Could you check a few things on this drawing? It's one solid part, dimensions in mm from its lowest x, y, z. A direction names the side the tool comes from. Give positions to 0.01 mm unless a question says otherwise; leave off trailing zeros. Loops run counter-clockwise (first coordinate to the right, second up) from the corner with the lowest first, then second, coordinate; pieces in that order, holes last.
1. I need wall thicknesses on line 1 along Z through (x, y) = (17.5, 22.75); line 2 along X through (y, z) = (18.25, 76.5) (1 decimal); line 3 along Y through (x, z) = (36.5, 49). Which ranges of each line are inside material? Lowest first, please.
2. Imagine slicing it at C-C (z = 34). List the corners of the cut face in (x, y) for me (1 decimal).
3. For P1, Ø3, axis at x = 61, z = 55.5, coming from the -Y side, with a flat end and sliding along its axis, tell me the tip position at first contact or that it passes through.
4. Imagine slicing it at B-B (y = 21). List the corners of the cut face in (x, z) for me (1 decimal), plus the area to 3 significant figures.
5. For the marked faces 1 and 2, which set-ups out of +Z, -Z, +X, -X, +Y, -Y let a thin tool reach every point of the face, with its end or its side?
6. Thinking about a two-plate mould opening in X: for the marked faces 3, 4 and 5, which applies, +X half, -X half, draft (parallel to the pull), parting line (faces both ways), or undercut?
7. Imagine slicing it at A-A (x = 61.5). List the corners of the cut face in (y, z) for me, plus the area to 3 significant figures.
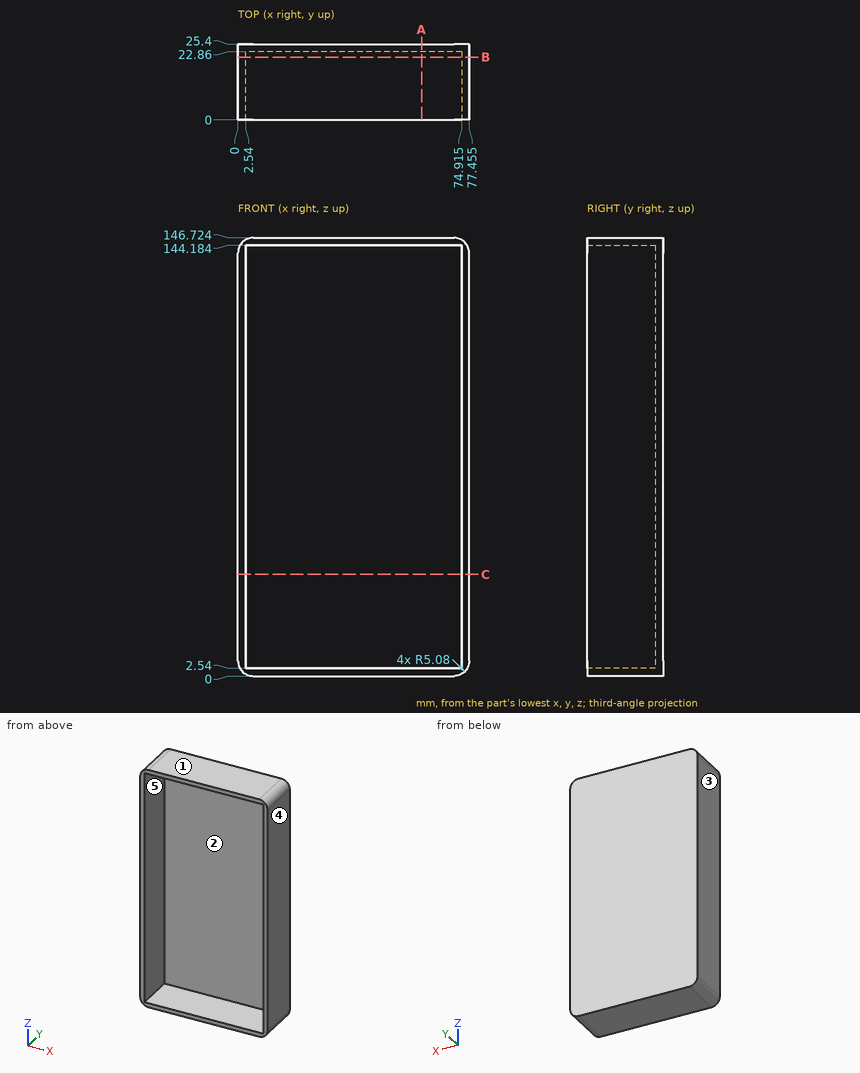
Derived:
1. line 1: z = 0 to 2.54, 144.18 to 146.72
1. line 2: x = 0 to 2.5, 74.9 to 77.5
1. line 3: y = 22.86 to 25.4
2. outline: (0, 0) - (2.5, 0) - (2.5, 22.9) - (74.9, 22.9) - (74.9, 0) - (77.5, 0) - (77.5, 25.4) - (0, 25.4) - close
3. P1: stops at y = 22.86
4. outline: (0, 5.1) arc R5.1 ccw to (5.1, 0) - (72.4, 0) arc R5.1 ccw to (77.5, 5.1) - (77.5, 141.6) arc R5.1 ccw to (72.4, 146.7) - (5.1, 146.7) arc R5.1 ccw to (0, 141.6) - close; hole (2.5, 2.5) - (74.9, 2.5) - (74.9, 144.2) - (2.5, 144.2) - close
4. area: 1,090 mm2
5. face 1: +Z, +X, -X, +Y, -Y
5. face 2: -Y
6. face 3: -X half
6. face 4: +X half
6. face 5: undercut
7. outline: (0, 0) - (25.4, 0) - (25.4, 146.72) - (0, 146.72) - (0, 144.18) - (22.86, 144.18) - (22.86, 2.54) - (0, 2.54) - close
7. area: 489 mm2
